```python
from build123d import *

# Parameters (mm, degrees)
F0_W      = 210
F0_H      = 180
F0_W_2    = 202
F0_H_2    = 40
F1_DEPTH  = 80
F2_W      = 4
F2_H      = 140
F3_DEPTH  = 2
F4_W      = 4
F4_H      = 140
F5_DEPTH  = 2
F6_W      = 2
F6_H      = 130
F7_DEPTH  = 2
F8_W      = 2
F8_H      = 130
F9_DEPTH  = 2
F11_DEPTH = 5


with BuildPart() as f1:
    # F0 (on Front) → F1 (new body)
    with BuildSketch(Plane.XZ):
        with Locations((-8.9074341967, -7.9735703766)):
            Rectangle(F0_W, F0_H)
        with Locations((-8.9074341967, -73.9735703766)):
            Rectangle(F0_W_2, F0_H_2, mode=Mode.SUBTRACT)
        with Locations((-8.9074341967, -29.9735703766)):
            Rectangle(F0_W_2, F0_H_2, mode=Mode.SUBTRACT)
        with Locations((-8.9074341967, 14.0264296234)):
            Rectangle(F0_W_2, F0_H_2, mode=Mode.SUBTRACT)
        with Locations((-8.9074341967, 58.0264296234)):
            Rectangle(F0_W_2, F0_H_2, mode=Mode.SUBTRACT)
    extrude(amount=F1_DEPTH)

    # F2 (on face) → F3 (join)
    with BuildSketch(Plane.YZ.offset(96.0925658033)):
        with Locations((2, -27.9735703766)):
            Rectangle(F2_W, F2_H)
    extrude(amount=-F3_DEPTH)

    # F4 (on face) → F5 (join)
    with BuildSketch(Plane(origin=(-113.9074341967, 0, 0), x_dir=(0, -1, 0), z_dir=(-1, 0, 0))):
        with Locations((-2, -27.9735703766)):
            Rectangle(F4_W, F4_H)
    extrude(amount=-F5_DEPTH)

    # F6 (on face) → F7 (join)
    with BuildSketch(Plane.YZ.offset(-111.9074341967)):
        with Locations((3, -32.9735703766)):
            Rectangle(F6_W, F6_H)
    extrude(amount=F7_DEPTH)

    # F8 (on face) → F9 (join)
    with BuildSketch(Plane(origin=(94.0925658033, 0, 0), x_dir=(0, -1, 0), z_dir=(-1, 0, 0))):
        with Locations((-3, -32.9735703766)):
            Rectangle(F8_W, F8_H)
    extrude(amount=F9_DEPTH)

    # F10 (on face) → F11 (join)
    with BuildSketch(Plane.XZ.offset(80)):
        Polygon((-109.9074341967, -45.9735703766), (-109.9074341967, -49.9735703766), (-105.9074341967, -49.9735703766), align=None)
        Polygon((-109.9074341967, -89.9735703766), (-109.9074341967, -93.9735703766), (-105.9074341967, -93.9735703766), align=None)
        Polygon((92.0925658033, -89.9735703766), (88.0925658033, -93.9735703766), (92.0925658033, -93.9735703766), align=None)
        Polygon((92.0925658033, -45.9735703766), (88.0925658033, -49.9735703766), (92.0925658033, -49.9735703766), align=None)
        Polygon((-109.9074341967, -1.9735703766), (-109.9074341967, -5.9735703766), (-105.9074341967, -5.9735703766), align=None)
        Polygon((92.0925658033, -1.9735703766), (88.0925658033, -5.9735703766), (92.0925658033, -5.9735703766), align=None)
        Polygon((92.0925658033, 42.0264296234), (88.0925658033, 38.0264296234), (92.0925658033, 38.0264296234), align=None)
        Polygon((-109.9074341967, 42.0264296234), (-109.9074341967, 38.0264296234), (-105.9074341967, 38.0264296234), align=None)
    extrude(amount=-F11_DEPTH)


solid = f1.part
```
Build history of the part. All positions in model axes, mm. A direction names the side the tool comes from. Give positions to 0.01 mm unless a question says otherwise; leave off trailing zeros. Loops run counter-clockwise (first coordinate to the right, second up) from the corner with the lowest first, then second, coordinate; pieces in that order, holes last.
Item 1: Drill centre lines: line 1 (Z direction, x = 54, y = -68.5); line 2 (X direction, y = -20, z = -79). Where is each one in solid material? Low to high.
Answers follow:
line 1: z = -97.97 to -93.97, -53.97 to -49.97, -9.97 to -5.97, 34.03 to 38.03, 78.03 to 82.03
line 2: x = -113.91 to -109.91, 92.09 to 96.09
Item 2: Which spindle directions (+Z, -Z, +X, -X, +Y, -Y) get a long thin tool onto all of the face, cutting with end or side? Do faces 4 (the face through (-10, -39, 78.026)), 5 (the face through (-33, -80, -8)). Say none if no direction does.
Answers follow:
face 4: +Y, -Y
face 5: +Z, -Z, +X, -X, -Y
Item 3: Slice it at A-A, the plane z = -80.5. List the corners of the cut face in (x, y).
Answers follow:
outline: (-113.91, -80) - (-109.91, -80) - (-109.91, 0) - (-111.91, 0) - (-111.91, 2) - (-109.91, 2) - (-109.91, 4) - (-113.91, 4) - close; (92.09, -80) - (96.09, -80) - (96.09, 4) - (92.09, 4) - (92.09, 2) - (94.09, 2) - (94.09, 0) - (92.09, 0) - close
Item 4: Slice it at C-C, the plane y = -69.5. List the corners of the cut face in (x, z).
Answers follow:
outline: (-113.91, -97.97) - (96.09, -97.97) - (96.09, 82.03) - (-113.91, 82.03) - close; hole (-109.91, -93.97) - (92.09, -93.97) - (92.09, -53.97) - (-109.91, -53.97) - close; hole (-109.91, -49.97) - (92.09, -49.97) - (92.09, -9.97) - (-109.91, -9.97) - close; hole (-109.91, -5.97) - (92.09, -5.97) - (92.09, 34.03) - (-109.91, 34.03) - close; hole (-109.91, 38.03) - (92.09, 38.03) - (92.09, 78.03) - (-109.91, 78.03) - close
Item 5: Slice it at B-B, the plane x = -56.5. List the corners of the cut face in (y, z).
Answers follow:
outline: (-80, -97.97) - (0, -97.97) - (0, -93.97) - (-80, -93.97) - close; (-80, -53.97) - (0, -53.97) - (0, -49.97) - (-80, -49.97) - close; (-80, -9.97) - (0, -9.97) - (0, -5.97) - (-80, -5.97) - close; (-80, 34.03) - (0, 34.03) - (0, 38.03) - (-80, 38.03) - close; (-80, 78.03) - (0, 78.03) - (0, 82.03) - (-80, 82.03) - close
Item 6: Slice it at D-D, the plane z = 48.5. List the corners of the cut face in (x, y).
Answers follow:
outline: (-113.91, -80) - (-109.91, -80) - (-109.91, 0) - (-113.91, 0) - close; (92.09, -80) - (96.09, -80) - (96.09, 0) - (92.09, 0) - close
Item 7: Flat gauge pin, fed straight in: pin 1 (4.5 mm diameter, centred on x = -107.5, z = 39.5, fed in from +Y). Where does the tip first touch, or does it go through?
Answers follow:
pin 1: stops at y = 0
Item 8: Pull direction X, two halves, no side cores. Call faces 1 (the face through (-113.907, -37, -7)), 2 (the face through (-10, -39, 82.026)), 3 (the face through (-10, -39, 38.026)): released by +X, released by -X, zero draft, split by the parting line, or undercut.
Answers follow:
face 1: released by -X
face 2: zero draft
face 3: undercut
